Source: CAD feature listing. Evaluate the final solid. Frame: model axes, mm. Face numbers are marked on the shaded views. Round coordinates to 2 decimals unless told otherwise and drop trailing zeros. Loops run counter-clockwise (first coordinate to the right, second up) from the corner with the lowest first, then second, coordinate; pieces in that order, holes last.
(1) First-contact query: pin 1 Ø7 at (x, y) = (30, -6) entering from -Z. Flat tip, straight axial feed; report the tip coordinate or a pass-through.
(2) Mould query, pull axis X, two halves, no side actions, for the marked faces 1, 2, 3 and 4. Classes: pulls with the +X half, pulls with the -X half, needs draft (parallel to the pull), parting line crosses it, or undercut.
(3) Material intervals for probe 1 along Y at (x, z) = (30, 1.75); probe 2 along Y at (x, z) = (31, 1.1); probe 3 along X at (y, z) = (6, 0.35), sorted ascending.
(4) Section A-A, the plane x = 30. Return the cut outline in (y, z), plus the area to 3 significant figures.
(5) Section D-D, the plane y = 3. Return the cut outline in (x, z), plus the area to 3 significant figures.
(6) Section C-C, the plane y = -6. Return the cut outline in (x, z), plus the area to 4 significant figures.
(7) Section B-B, the plane z = 2.7. Return the cut outline in (x, y).
```python
from build123d import *

# Parameters (mm, degrees)
SKETCH1_W               = 40
SKETCH1_H               = 25
BOSS_EXTRUDE1_DEPTH     = 4
SKETCH7_W               = 9
SKETCH7_H               = 25
CUT_EXTRUDE5_DEPTH      = 21
SKETCH8_W               = 20
SKETCH8_H               = 25
BOSS_EXTRUDE2_DEPTH     = 4
CUT_EXTRUDE6_DEPTH      = 43.09809972
CUT_EXTRUDE6_DEPTH_BACK = 43.09809972
SKETCH9_R               = 2.5
CUT_EXTRUDE7_DEPTH      = 0.5
FILLET1_R               = 1
SKETCH11_W              = 20
SKETCH11_H              = 25
CUT_EXTRUDE8_DEPTH      = 10


with BuildPart() as part:
    # Sketch1 → Boss-Extrude1 (new body)
    with BuildSketch(Plane.XY):
        Rectangle(SKETCH1_W, SKETCH1_H)
    extrude(amount=BOSS_EXTRUDE1_DEPTH)

    # Sketch7 → Cut-Extrude5 (cut)
    with BuildSketch(Plane.XY):
        with Locations((-15.5, 0)):
            Rectangle(SKETCH7_W, SKETCH7_H)
    extrude(amount=CUT_EXTRUDE5_DEPTH, mode=Mode.SUBTRACT)

    # Sketch8 → Boss-Extrude2 (add)
    with BuildSketch(Plane.XY):
        with Locations((30, 0)):
            Rectangle(SKETCH8_W, SKETCH8_H)
    extrude(amount=BOSS_EXTRUDE2_DEPTH)

    # Sketch9 → Cut-Extrude6 (cut, two sides: drawn at the far end of the back side and taken through both)
    with BuildSketch(Plane.XY.offset(-CUT_EXTRUDE6_DEPTH_BACK)):
        with Locations(Location((30, 6, 0), (0, 0, 180))):
            Circle(SKETCH9_R)
        with Locations(Location((30, -6, 0), (0, 0, 180))):
            Circle(SKETCH9_R)
    extrude(amount=CUT_EXTRUDE6_DEPTH + CUT_EXTRUDE6_DEPTH_BACK, mode=Mode.SUBTRACT)

    # Sketch10 → Cut-Extrude7 (cut)
    with BuildSketch(Plane.XY):
        with BuildLine():
            Line((32.705156976, 0.644430401), (32.705156976, -0.644430401))
            ThreePointArc((32.705156976, -0.644430401), (29.983190138, -11.999976452), (27.324894168, -0.629356762))
            Line((27.324894168, -0.629356762), (27.324894168, 0.629356762))
            ThreePointArc((27.324894168, 0.629356762), (29.983190138, 11.999976452), (32.705156976, 0.644430401))
        make_face()
    extrude(amount=CUT_EXTRUDE7_DEPTH, mode=Mode.SUBTRACT)

    # Fillet1
    fillet1_edges = [part.edges().sort_by_distance(p)[0] for p in [
        (27.324894168, 0.629356762, 0.25),
        (27.324894168, -0.629356762, 0.25),
        (32.705156976, -0.644430401, 0.25),
        (32.705156976, 0.644430401, 0.25),
    ]]
    fillet(fillet1_edges, radius=FILLET1_R)

    # Sketch11 → Cut-Extrude8 (cut)
    with BuildSketch(Plane.XY):
        with Locations((-1, 0)):
            Rectangle(SKETCH11_W, SKETCH11_H)
    extrude(amount=CUT_EXTRUDE8_DEPTH, mode=Mode.SUBTRACT)


solid = part.part
```
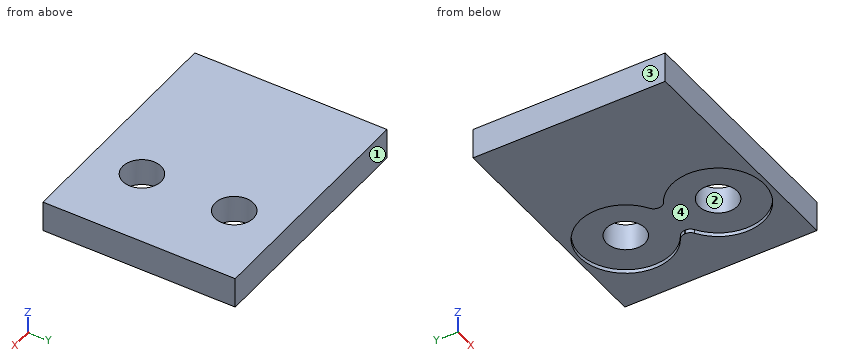
Output values:
1. pin 1: stops at z = 0.5
2. face 1: needs draft
2. face 2: undercut
2. face 3: pulls with the -X half
2. face 4: undercut
3. probe 1: y = -12.5 to -8.5, -3.5 to 3.5, 8.5 to 12.5
3. probe 2: y = -12.5 to -8.29, -3.71 to 3.71, 8.29 to 12.5
3. probe 3: x = 9 to 24, 36 to 40
4. outline: (-12.5, 0) - (-12, 0) - (-12, 0.5) - (-8.5, 0.5) - (-8.5, 4) - (-12.5, 4) - close; (-3.5, 0.5) - (3.5, 0.5) - (3.5, 4) - (-3.5, 4) - close; (8.5, 0.5) - (12, 0.5) - (12, 0) - (12.5, 0) - (12.5, 4) - (8.5, 4) - close
4. area: 53.0 mm2
5. outline: (9, 0) - (24.8, 0) - (24.8, 0.5) - (35.2, 0.5) - (35.2, 0) - (40, 0) - (40, 4) - (9, 4) - close
5. area: 119 mm2
6. outline: (9, 0) - (24, 0) - (24, 0.5) - (27.5, 0.5) - (27.5, 4) - (9, 4) - close; (32.5, 0.5) - (36, 0.5) - (36, 0) - (40, 0) - (40, 4) - (32.5, 4) - close
6. area: 100.5 mm2
7. outline: (9, -12.5) - (40, -12.5) - (40, 12.5) - (9, 12.5) - close; hole circle Ø5 at (30, -6); hole circle Ø5 at (30, 6)
